Autodesk Fusion 360 part; units mm, degrees
sketch "Sketch2" plane through (0, 0, 0) normal (0, 0, 1) x (1, 0, 0)
  line L0 (0, 0) -> (6, 0)
  line L1 (0, 0) -> (0, 6)
  line L2 (0, 6) -> (6, 6)
  line L3 (6, 6) -> (6, 0)
  circle A0 centre (3, 3) radius 1.9
  circle A1 centre (3, 3) radius 0.95
  dimension "d11" = 6
  dimension "d12" = 6
  dimension "d13" = 6
  dimension "d15" = 3.8
  dimension "d16" = 1.9
extrude "Extrude4" add sketch "Sketch2" along normal blind 3 contours A0
extrude "Extrude5" add sketch "Sketch2" along normal blind 1 contours L0 L1 L2 L3
extrude "Extrude6" add sketch "Sketch2" along normal blind 1 contours A1
CAD build for the part. Positions are in the model's coordinates, mm. A direction names the side the tool comes from. Round coordinates to 2 decimals unless told otherwise and drop trailing zeros. Write each loop counter-clockwise with the first axis right and the second up, starting at its lowest first coordinate (ties: lowest second). Pieces come first, ordered by that corner, then holes.
(1) Slice it at D-D, the plane x = 4.35. Write the cut outline in (y, z), and give its area (3 significant figures).
(2) Slice it at C-C, the plane z = 2.8. Write the cut outline in (x, y), and give its area (3 significant figures).
(3) Probe line 1 along Y through (x, z) = (3, 1.75); line 2 along Z through (x, y) = (5.45, 4.85); line 3 along Y through (x, z) = (3.8, 2.2). List the from-to ranges inside material, lowest first.
(4) 3-axis set-ups, long thin cutter, end or side, ignore diameter. For faces 4 (the face through (3, 6, 0.5)), 5 (the face through (4.021, 1.398, 1.986)): which of +Z, -Z, +X, -X, +Y, -Y reach the whole face in a straight line?
(5) Drop flat-ended pins along their axis: P1, Ø1.7, axis at x = 3, y = 3, coming from the -Z side; P2, Ø0.6, axis at x = 3.5, y = 3, coming from the +Z side. Give the stop position or say it passes through.
(6) Slice it at A-A, the plane y = 3. Write the cut outline in (x, z), and give its area (3 significant figures).
(7) Mould opens along X. For faces 1 (the face through (0, 3, 0.5)), 2 (the face through (3, 3, 1)), 3 (the face through (3, 0, 0.5)) say: pulls with the +X half, pulls with the -X half, needs draft (parallel to the pull), parting line crosses it, or undercut.
From the geometry:
1. outline: (0, 0) - (6, 0) - (6, 1) - (4.34, 1) - (4.34, 3) - (1.66, 3) - (1.66, 1) - (0, 1) - close
1. area: 11.3 mm2
2. outline: circle Ø3.8 at (3, 3); hole circle Ø1.9 at (3, 3)
2. area: 8.51 mm2
3. line 1: y = 1.1 to 2.05, 3.95 to 4.9
3. line 2: z = 0 to 1
3. line 3: y = 1.28 to 2.49, 3.51 to 4.72
4. face 4: +Z, -Z, +X, -X, +Y
4. face 5: +Z
5. P1: stops at z = 0
5. P2: stops at z = 1
6. outline: (0, 0) - (6, 0) - (6, 1) - (4.9, 1) - (4.9, 3) - (3.95, 3) - (3.95, 1) - (2.05, 1) - (2.05, 3) - (1.1, 3) - (1.1, 1) - (0, 1) - close
6. area: 9.80 mm2
7. face 1: pulls with the -X half
7. face 2: undercut
7. face 3: needs draft
